The drawing under review shows one solid part. Ordinate dimensions are in mm from its lowest x, y, z. Round coordinates to 2 decimals unless told otherwise and drop trailing zeros. Write each loop counter-clockwise with the first axis right and the second up, starting at its lowest first coordinate (ties: lowest second). Pieces come first, ordered by that corner, then holes. Notation, with made-up numbers: (31.5, 12) -> (41.5, 12) arc R5 ccw to (41.5, 17) -> close; hole circle Ø9 at (65.25, 48.25). An arc over 180 degrees is marked (long way). Answer in a Markdown table with one row per item.
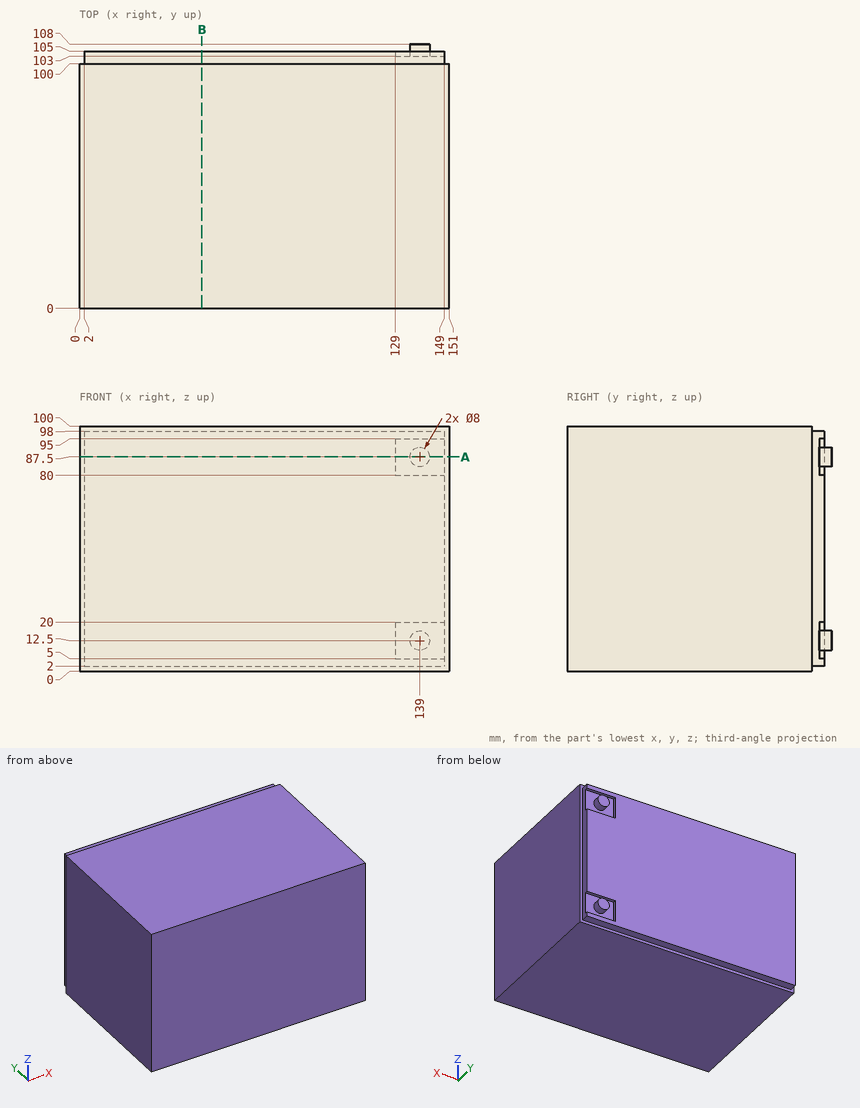
1) Clearance check with flat-ended pins moving along their axes: pin 1 Ø4 at (y, z) = (103.5, 55) entering from -X; pin 2 Ø4 at (y, z) = (102.5, 71) entering from +X; pin 3 Ø1.6 at (x, y) = (134.5, 103.5) entering from -Z. State where each tip first meets the part, or that it passes through.
Solved:
| item | result |
|---|---|
| pin 1 | x = 2 |
| pin 2 | x = 149 |
| pin 3 | z = 2 |
2) Consider section A-A on z = 87.5. State the section outline as (x, y) points, then the cut area to 3 significant figures.
Solved:
| item | result |
|---|---|
| outline | (0, 0) -> (151, 0) -> (151, 100) -> (149, 100) -> (149, 103) -> (143, 103) -> (143, 108) -> (135, 108) -> (135, 103) -> (129, 103) -> (129, 105) -> (2, 105) -> (2, 100) -> (0, 100) -> close |
| area | 15,800 mm² |
3) For line 1 (Y direction, x = 119, z = 16), list the stretches that pass through material, from the lowest coordinate up. Write a range as [from, to].
Solved:
| item | result |
|---|---|
| line 1 | [0, 105] |
4) Consider section B-B on x = 50. State the section outline as (y, z) points, then the cut area to 3 significant figures.
Solved:
| item | result |
|---|---|
| outline | (0, 0) -> (100, 0) -> (100, 2) -> (105, 2) -> (105, 98) -> (100, 98) -> (100, 100) -> (0, 100) -> close |
| area | 10,500 mm² |
